```python
from build123d import *

# Parameters (mm, degrees)
SKETCH1_R           = 2.5
BOSS_EXTRUDE1_DEPTH = 3


with BuildPart() as part:
    # Sketch1 → Boss-Extrude1 (new body)
    with BuildSketch(Plane(origin=(0, 0, 0), x_dir=(1, 0, 0), z_dir=(0, 1, 0))):
        Polygon((59.8, 97), (40, 97), (40, 100), (19.8, 100), (19.8, 97), (3, 97), (3, 80.2), (0, 80.2), (0, 60), (3, 60), (3, 40.2), (0, 40.2), (0, 20), (3, 20), (3, 3), (19.8, 3), (19.8, 0), (40, 0), (40, 3), (59.8, 3), (59.8, 0), (80, 0), (80, 3), (97, 3), (97, 20), (100, 20), (100, 40.2), (97, 40.2), (97, 60), (100, 60), (100, 80.2), (97, 80.2), (97, 97), (80, 97), (80, 100), (59.8, 100), align=None)
        with Locations((50, 50)):
            Circle(SKETCH1_R, mode=Mode.SUBTRACT)
    extrude(amount=BOSS_EXTRUDE1_DEPTH)


solid = part.part
```
Could you check a few things on this model? Use its own coordinates, in mm. A direction names the side the tool comes from. Coordinates: 2 decimals unless noted, no trailing zeros. Write each loop counter-clockwise with the first axis right and the second up, starting at its lowest first coordinate (ties: lowest second). Pieces come first, ordered by that corner, then holes. Notation, with made-up numbers: (13, 51) - (66, 51) arc R22 cw to (66, 65) - close; hole circle Ø10 at (85, 36). An arc over 180 degrees is marked (long way). Use a Markdown table: item, result.
Q1. Which directions (+Z, -Z, +X, -X, +Y, -Y) give clear straight access to the entire face, cutting with the end or side of a thin tool? Please do faces 4 (the flat face through (50, 1, -3)), 5 (the flat face through (11, 1, -3)), 6 (the flat face through (50, 1, -97)).
Geometry check:
| item | result |
|---|---|
| face 4 | +Z, +Y, -Y |
| face 5 | +Z, -X, +Y, -Y |
| face 6 | -Z, +Y, -Y |
Q2. Imagine slicing it at D-D (z = -13.5). List the corners of the cut face in (x, y) for me.
Geometry check:
| item | result |
|---|---|
| outline | (3, 0) - (97, 0) - (97, 3) - (3, 3) - close |
Q3. Imagine slicing it at B-B (z = -50). List the corners of the cut face in (x, y) for me, and give its area (3 significant figures).
Geometry check:
| item | result |
|---|---|
| outline | (3, 0) - (47.5, 0) - (47.5, 3) - (3, 3) - close; (52.5, 0) - (97, 0) - (97, 3) - (52.5, 3) - close |
| area | 267 mm2 |
Q4. I'm going to push flat-ended pins straight in: pin 1 Ø1.5 at (x, y) = (51.5, 1) entering from +Z; pin 2 Ø1.5 at (y, z) = (2, -2) entering from +X; pin 3 Ø3 at (x, z) = (50, -50) entering from +Y; pin 4 Ø0.9 at (y, z) = (1.5, -92.5) entering from +X. Where does each tip first touch, or does it pass through?
Geometry check:
| item | result |
|---|---|
| pin 1 | stops at z = -3 |
| pin 2 | stops at x = 80 |
| pin 3 | passes through |
| pin 4 | stops at x = 97 |
Q5. Please list where these lines run through material, in increasing order: L1, parallel to X at y = 1.3, z = -50; L2, parallel to Z at x = 50, y = 1.25; L3, parallel to X at y = 0.9, z = -55.
Geometry check:
| item | result |
|---|---|
| L1 | x = 3 to 47.5, 52.5 to 97 |
| L2 | z = -97 to -52.5, -47.5 to -3 |
| L3 | x = 3 to 97 |
Q6. Thinking about a two-plate mould opening in X: for faces 1 (the flat face through (3, 1, -12)), 2 (the flat face through (70, 1, 0)), 3 (the flat face through (59.8, 1, -2)), which applies, +X half, -X half, draft (parallel to the pull), parting line (faces both ways), or undercut?
Geometry check:
| item | result |
|---|---|
| face 1 | -X half |
| face 2 | draft |
| face 3 | undercut |
Q7. Imagine slicing it at C-C (x = 16). List the corners of the cut face in (y, z) for me.
Geometry check:
| item | result |
|---|---|
| outline | (0, -97) - (3, -97) - (3, -3) - (0, -3) - close |
Q8. Imagine slicing it at A-A (x = 50). List the corners of the cut face in (y, z) for me, and give its area (3 significant figures).
Geometry check:
| item | result |
|---|---|
| outline | (0, -97) - (3, -97) - (3, -52.5) - (0, -52.5) - close; (0, -47.5) - (3, -47.5) - (3, -3) - (0, -3) - close |
| area | 267 mm2 |
